Design review of the part built by this model. Coordinates are the model's own, in mm. Coordinates: 2 decimals unless noted, no trailing zeros.
Q1. The part is to be moulded in two halves that separate along X. For faces 1 (the face through (-1.83, -8.58, 98.6)), 2 (the face through (-8, 3.9, 99)), 3 (the face through (-11.504, -13, 99)), say which applies: +X half, -X half, draft (parallel to the pull), parting line (faces both ways), or undercut.
Q2. Clearance check with flat-ended pins moving along their axes: pin 1 Ø2.5 at (y, z) = (-6.5, 52) entering from +X; pin 2 Ø0.9 at (x, z) = (-2, 55.5) entering from -Y. State where each tip first meets the part, or that it passes through.
Q3. To check wall thickness, follow probe 1 along X at (y, z) = (-14.25, 40.5); probe 2 along Y at (x, z) = (5.5, 100.5); probe 3 along Y at (x, z) = (-10.25, 56). State the ranges of each line that lie inside material, in increasing order.
Autodesk Inventor part; units mm, degrees
ref_plane "YZ Plane" through (0, 0, 0) normal (1, 0, 0) x (0, 1, 0)
ref_plane "XZ Plane" through (0, 0, 0) normal (0, 1, 0) x (-1, 0, 0)
ref_plane "XY Plane" through (0, 0, 0) normal (0, 0, 1) x (1, 0, 0)
sketch "Sketch1" plane through (0, 0, 0) normal (0, 0, 1) x (1, 0, 0)
  line L0 (1.7678, -1.7678) -> (3.9962, 0.4607)
  arc A0 (0, -2.5) -> (1.7678, -1.7678) centre (0, 0) ccw
  line L1 (-3.0076, -2.5) -> (0, -2.5)
  arc A1 (-4.7754, -1.7678) -> (-3.0076, -2.5) centre (-3.0076, 0) ccw
  line L2 (-7.0038, 0.4607) -> (-4.7754, -1.7678)
  line L3 (-7.0038, 2.4) -> (-7.0038, 0.4607)
  line L4 (-5.0038, 2.4) -> (-7.0038, 2.4)
  arc A2 (-5.0038, 2.4) -> (-4.6038, 2.8) centre (-5.0038, 2.8) ccw
  line L5 (-5.7038, 3.9) -> (-4.6038, 2.8)
  line L6 (-11.1038, 3.9) -> (-5.7038, 3.9)
  arc A3 (-11.1038, 3.9) -> (-11.5038, 3.5) centre (-11.1038, 3.5) ccw
  line L7 (-11.5038, -1.9) -> (-11.5038, 3.5)
  line L8 (-10.4038, -3) -> (-11.5038, -1.9)
  arc A4 (-10.4038, -3) -> (-10.0038, -2.6) centre (-10.4038, -2.6) ccw
  line L9 (-10.0038, -0.6) -> (-10.0038, -2.6)
  line L10 (-8.0645, -0.6) -> (-10.0038, -0.6)
  line L11 (-5.836, -2.8284) -> (-8.0645, -0.6)
  arc A5 (-5.1038, -4.5962) -> (-5.836, -2.8284) centre (-7.6038, -4.5962) ccw
  line L12 (-5.1038, -7.6038) -> (-5.1038, -4.5962)
  arc A6 (-5.836, -9.3716) -> (-5.1038, -7.6038) centre (-7.6038, -7.6038) ccw
  line L13 (-8.0645, -11.6) -> (-5.836, -9.3716)
  line L14 (-10.0038, -11.6) -> (-8.0645, -11.6)
  line L15 (-10.0038, -9.6) -> (-10.0038, -11.6)
  arc A7 (-10.0038, -9.6) -> (-10.4038, -9.2) centre (-10.4038, -9.6) ccw
  line L16 (-11.5038, -10.3) -> (-10.4038, -9.2)
  line L17 (-11.5038, -15.7) -> (-11.5038, -10.3)
  arc A8 (-11.5038, -15.7) -> (-11.1038, -16.1) centre (-11.1038, -15.7) ccw
  line L18 (-5.7038, -16.1) -> (-11.1038, -16.1)
  line L19 (-4.6038, -15) -> (-5.7038, -16.1)
  arc A9 (-4.6038, -15) -> (-5.0038, -14.6) centre (-5.0038, -15) ccw
  line L20 (-7.0038, -14.6) -> (-5.0038, -14.6)
  line L21 (-7.0038, -12.6607) -> (-7.0038, -14.6)
  line L22 (-4.7754, -10.4322) -> (-7.0038, -12.6607)
  arc A10 (-3.0076, -9.7) -> (-4.7754, -10.4322) centre (-3.0076, -12.2) ccw
  line L23 (0, -9.7) -> (-3.0076, -9.7)
  arc A11 (1.7678, -10.4322) -> (0, -9.7) centre (0, -12.2) ccw
  line L24 (3.9962, -12.6607) -> (1.7678, -10.4322)
  line L25 (3.9962, -14.6) -> (3.9962, -12.6607)
  line L26 (1.9962, -14.6) -> (3.9962, -14.6)
  arc A12 (1.9962, -14.6) -> (1.5962, -15) centre (1.9962, -15) ccw
  line L27 (2.6962, -16.1) -> (1.5962, -15)
  line L28 (8.0962, -16.1) -> (2.6962, -16.1)
  arc A13 (8.0962, -16.1) -> (8.4962, -15.7) centre (8.0962, -15.7) ccw
  line L29 (8.4962, -10.3) -> (8.4962, -15.7)
  line L30 (7.3962, -9.2) -> (8.4962, -10.3)
  arc A14 (7.3962, -9.2) -> (6.9962, -9.6) centre (7.3962, -9.6) ccw
  line L31 (6.9962, -11.6) -> (6.9962, -9.6)
  line L32 (5.0569, -11.6) -> (6.9962, -11.6)
  line L33 (2.8284, -9.3716) -> (5.0569, -11.6)
  arc A15 (2.0962, -7.6038) -> (2.8284, -9.3716) centre (4.5962, -7.6038) ccw
  line L34 (2.0962, -4.5962) -> (2.0962, -7.6038)
  arc A16 (2.8284, -2.8284) -> (2.0962, -4.5962) centre (4.5962, -4.5962) ccw
  line L35 (5.0569, -0.6) -> (2.8284, -2.8284)
  line L36 (6.9962, -0.6) -> (5.0569, -0.6)
  line L37 (6.9962, -2.6) -> (6.9962, -0.6)
  arc A17 (6.9962, -2.6) -> (7.3962, -3) centre (7.3962, -2.6) ccw
  line L38 (8.4962, -1.9) -> (7.3962, -3)
  line L39 (8.4962, 3.5) -> (8.4962, -1.9)
  arc A18 (8.4962, 3.5) -> (8.0962, 3.9) centre (8.0962, 3.5) ccw
  line L40 (2.6962, 3.9) -> (8.0962, 3.9)
  line L41 (1.5962, 2.8) -> (2.6962, 3.9)
  arc A19 (1.5962, 2.8) -> (1.9962, 2.4) centre (1.9962, 2.8) ccw
  line L42 (3.9962, 2.4) -> (1.9962, 2.4)
  line L43 (3.9962, 0.4607) -> (3.9962, 2.4)
  circle A20 centre (-1.5038, -6.1) radius 2.5
  point P0 (0, 0)
extrude "Extrusion1" add sketch "Sketch1" along normal blind 200
properties part number "00_VSlot_20mm"
Here are the results:
1. face 1: undercut
1. face 2: draft
1. face 3: -X half
2. pin 1: stops at x = 2.1
2. pin 2: stops at y = -9.7
3. probe 1: x = -11.5 to -7, 4 to 8.5
3. probe 2: y = -16.1 to -11.6, -0.6 to 3.9
3. probe 3: y = -16.1 to -9.23, -2.97 to 3.9
